from build123d import *

# Parameters (mm, degrees)
SKETCH1_W           = 16
SKETCH1_H           = 80
SKETCH1_R           = 1.625
BOSS_EXTRUDE1_DEPTH = 5
SKETCH2_R           = 1.75
BOSS_EXTRUDE2_DEPTH = 5


with BuildPart() as part:
    # Sketch1 → Boss-Extrude1 (new body)
    with BuildSketch(Plane.XY):
        with Locations((8, 40)):
            Rectangle(SKETCH1_W, SKETCH1_H)
        with Locations((8, 20)):
            Circle(SKETCH1_R, mode=Mode.SUBTRACT)
        with Locations((8, 60)):
            Circle(SKETCH1_R, mode=Mode.SUBTRACT)
        with BuildLine():
            Line((6.5, 50.5), (9.5, 50.5))
            ThreePointArc((9.5, 50.5), (10.75, 49.25), (9.5, 48))
            Line((9.5, 48), (6.5, 48))
            ThreePointArc((6.5, 48), (5.25, 49.25), (6.5, 50.5))
        make_face(mode=Mode.SUBTRACT)
        with BuildLine():
            Line((6.5, 43), (9.5, 43))
            ThreePointArc((9.5, 43), (10.75, 41.75), (9.5, 40.5))
            Line((9.5, 40.5), (6.5, 40.5))
            ThreePointArc((6.5, 40.5), (5.25, 41.75), (6.5, 43))
        make_face(mode=Mode.SUBTRACT)
    extrude(amount=BOSS_EXTRUDE1_DEPTH)

    # Sketch2 → Boss-Extrude2 (add)
    # profile 1 of 2: a face of its own
    with BuildSketch(Plane.XY.offset(5)):
        with BuildLine():
            Line((16, 80), (23, 80))
            ThreePointArc((23, 80), (25.121320344, 79.121320344), (26, 77))
            Line((26, 77), (26, 3))
            ThreePointArc((26, 3), (25.121320344, 0.878679656), (23, 0))
            Line((23, 0), (16, 0))
            Line((16, 0), (16, 80))
        make_face()
        with Locations((21, 70)):
            Circle(SKETCH2_R, mode=Mode.SUBTRACT)
        with Locations((21, 65)):
            Circle(SKETCH2_R, mode=Mode.SUBTRACT)
        with Locations((21, 60)):
            Circle(SKETCH2_R, mode=Mode.SUBTRACT)
        with Locations((21, 55)):
            Circle(SKETCH2_R, mode=Mode.SUBTRACT)
        with Locations((21, 50)):
            Circle(SKETCH2_R, mode=Mode.SUBTRACT)
        with Locations((21, 45)):
            Circle(SKETCH2_R, mode=Mode.SUBTRACT)
        with Locations((21, 40)):
            Circle(SKETCH2_R, mode=Mode.SUBTRACT)
        with Locations((21, 35)):
            Circle(SKETCH2_R, mode=Mode.SUBTRACT)
        with Locations((21, 30)):
            Circle(SKETCH2_R, mode=Mode.SUBTRACT)
        with Locations((21, 25)):
            Circle(SKETCH2_R, mode=Mode.SUBTRACT)
        with Locations((21, 20)):
            Circle(SKETCH2_R, mode=Mode.SUBTRACT)
        with Locations((21, 15)):
            Circle(SKETCH2_R, mode=Mode.SUBTRACT)
        with Locations((21, 10)):
            Circle(SKETCH2_R, mode=Mode.SUBTRACT)
    # profile 2 of 2: a face of its own
    with BuildSketch(Plane.XY.offset(5)):
        with BuildLine():
            Line((0, 0), (0, 80))
            Line((0, 80), (-7, 80))
            ThreePointArc((-7, 80), (-9.121320344, 79.121320344), (-10, 77))
            Line((-10, 77), (-10, 3))
            ThreePointArc((-10, 3), (-9.121320344, 0.878679656), (-7, 0))
            Line((-7, 0), (0, 0))
        make_face()
        with Locations(Location((-5, 10, 0), (0, 0, 180))):
            Circle(SKETCH2_R, mode=Mode.SUBTRACT)
        with Locations(Location((-5, 15, 0), (0, 0, 180))):
            Circle(SKETCH2_R, mode=Mode.SUBTRACT)
        with Locations(Location((-5, 20, 0), (0, 0, 180))):
            Circle(SKETCH2_R, mode=Mode.SUBTRACT)
        with Locations(Location((-5, 25, 0), (0, 0, 180))):
            Circle(SKETCH2_R, mode=Mode.SUBTRACT)
        with Locations(Location((-5, 30, 0), (0, 0, 180))):
            Circle(SKETCH2_R, mode=Mode.SUBTRACT)
        with Locations(Location((-5, 35, 0), (0, 0, 180))):
            Circle(SKETCH2_R, mode=Mode.SUBTRACT)
        with Locations(Location((-5, 40, 0), (0, 0, 180))):
            Circle(SKETCH2_R, mode=Mode.SUBTRACT)
        with Locations(Location((-5, 45, 0), (0, 0, 180))):
            Circle(SKETCH2_R, mode=Mode.SUBTRACT)
        with Locations(Location((-5, 50, 0), (0, 0, 180))):
            Circle(SKETCH2_R, mode=Mode.SUBTRACT)
        with Locations(Location((-5, 55, 0), (0, 0, 180))):
            Circle(SKETCH2_R, mode=Mode.SUBTRACT)
        with Locations(Location((-5, 60, 0), (0, 0, 180))):
            Circle(SKETCH2_R, mode=Mode.SUBTRACT)
        with Locations(Location((-5, 65, 0), (0, 0, 180))):
            Circle(SKETCH2_R, mode=Mode.SUBTRACT)
        with Locations(Location((-5, 70, 0), (0, 0, 180))):
            Circle(SKETCH2_R, mode=Mode.SUBTRACT)
    extrude(amount=-BOSS_EXTRUDE2_DEPTH)


solid = part.part
Design review of the part built by this model. Coordinates are the model's own, in mm. A direction names the side the tool comes from. Give positions to 0.01 mm unless a question says otherwise; leave off trailing zeros. Loops run counter-clockwise (first coordinate to the right, second up) from the corner with the lowest first, then second, coordinate; pieces in that order, holes last. Notation, with made-up numbers: M 43,55.25 L 94,55.25 A6 cw 94,62.25 Z; hole C 58,-10 d1. An arc over 180 degrees is marked long. Write item = value, one per line.
Q1. For faces 1 (the flat face through (8, 43, 2)), 2 (the flat face through (-10, 41, 3)), list the 3-axis set-ups (+Z, -Z, +X, -X, +Y, -Y) from which the entire face can be reached by the end or side of a thin tool; tool diameter is ignored.
Output values:
face_1 = +Z, -Z
face_2 = +Z, -Z, -X, +Y, -Y
Q2. Draft analysis for pull direction X (two halves, no side actions). For faces 3 (the cylindrical face through (-4.62, 66.71, 2.54)), 4 (the cylindrical face through (25.14, 0.9, 2.54)), 5 (the cylindrical face through (-9.1, 79.14, 2.54)), state which applies: +X half, -X half, draft (parallel to the pull), parting line (faces both ways), or undercut.
Output values:
face_3 = undercut
face_4 = +X half
face_5 = -X half
Q3. We need section B-B (y = 49.25). Give the boundary of the cut face in (x, z), plus the area to 3 significant figures.
Output values:
outline = M -10,0 L -6.58,0 L -6.58,5 L -10,5 Z; M -3.42,0 L 5.25,0 L 5.25,5 L -3.42,5 Z; M 10.75,0 L 19.42,0 L 19.42,5 L 10.75,5 Z; M 22.58,0 L 26,0 L 26,5 L 22.58,5 Z
area = 121 mm^2
Q4. We need section A-A (y = 65). Give the boundary of the cut face in (x, z), plus the area to 3 significant figures.
Output values:
outline = M -10,0 L -6.75,0 L -6.75,5 L -10,5 Z; M -3.25,0 L 19.25,0 L 19.25,5 L -3.25,5 Z; M 22.75,0 L 26,0 L 26,5 L 22.75,5 Z
area = 145 mm^2
Q5. To check wall thickness, follow line 1 (X direction, y = 65, z = 2.25); line 2 (X direction, y = 14, z = 2.55); line 3 (Y direction, x = 8.5, z = 2.3). State the ranges of each line that lie inside material, in increasing order. Write a range as [from, to].
Output values:
line_1 = [-10, -6.75], [-3.25, 19.25], [22.75, 26]
line_2 = [-10, -6.44], [-3.56, 19.56], [22.44, 26]
line_3 = [0, 18.45], [21.55, 40.5], [43, 48], [50.5, 58.45], [61.55, 80]
Q6. Insertion check: pin 1 (3 mm diameter, centred on x = 21, y = 70, fed in from -Z). The pin has a flat end and moves straight along its axis. Give the tip position at first contact, or say it passes through.
Output values:
pin_1 = through
Q7. We need section C-C (z = 2.65). Count the separate pieces of the cut face and the enclosed holes in it, plus the area to 3 significant figures.
Output values:
separate_pieces = 1
enclosed_holes = 30
area = 2,580 mm^2
